from build123d import *

# Parameters (mm, degrees)
SKETCH2_R           = 50
BOSS_EXTRUDE1_DEPTH = 3
SKETCH3_R           = 6
BOSS_EXTRUDE2_DEPTH = 38.1
FILLET1_R           = 6
CUT_EXTRUDE1_DEPTH  = 38.1
SKETCH7_R           = 1.1
CUT_EXTRUDE2_DEPTH  = 2.2
SKETCH8_R           = 1.5
CUT_EXTRUDE3_DEPTH  = 3


with BuildPart() as part:
    # Sketch2 → Boss-Extrude1 (new body)
    with BuildSketch(Plane(origin=(0, 0, 0), x_dir=(1, 0, 0), z_dir=(0, 1, 0))):
        with Locations(Location((0, 0, 0), (0, 0, 270))):
            Circle(SKETCH2_R)
    extrude(amount=BOSS_EXTRUDE1_DEPTH)

    # Sketch3 → Boss-Extrude2 (add)
    with BuildSketch(Plane(origin=(0, 3, 0), x_dir=(1, 0, 0), z_dir=(0, 1, 0))):
        with Locations(Location((0, 35, 0), (0, 0, 90))):
            Circle(SKETCH3_R)
    extrude(amount=BOSS_EXTRUDE2_DEPTH)

    # Fillet1
    fillet1_edges = [part.edges().sort_by_distance(p)[0] for p in [
        (0, 41.1, -29),
    ]]
    fillet(fillet1_edges, radius=FILLET1_R)

    # Sketch6 → Cut-Extrude1 (cut)
    with BuildSketch(Plane(origin=(0, 3, 0), x_dir=(1, 0, 0), z_dir=(0, 1, 0))):
        Polygon((-43.65, 24.386010334), (-43.65, -24.386010334), (-50, -24.386010334), (-50, 0), (-50, 24.386010334), align=None)
        Polygon((43.65, 24.386010334), (43.65, -24.386010334), (50, -24.386010334), (50, 0), (50, 24.386010334), align=None)
    extrude(amount=-CUT_EXTRUDE1_DEPTH, mode=Mode.SUBTRACT)

    # Sketch7 → Cut-Extrude2 (cut)
    with BuildSketch(Plane(origin=(0, 3, 0), x_dir=(1, 0, 0), z_dir=(0, 1, 0))):
        with Locations(Location((-28.93, 11.280989666, 0), (0, 0, 270))):
            Circle(SKETCH7_R)
        with Locations(Location((-18.77, 11.280989666, 0), (0, 0, 270))):
            Circle(SKETCH7_R)
        with Locations(Location((19.07, 11.280989666, 0), (0, 0, 270))):
            Circle(SKETCH7_R)
        with Locations(Location((29.23, 11.280989666, 0), (0, 0, 270))):
            Circle(SKETCH7_R)
        with Locations(Location((29.23, -32.153010334, 0), (0, 0, 270))):
            Circle(SKETCH7_R)
        with Locations(Location((19.07, -32.153010334, 0), (0, 0, 270))):
            Circle(SKETCH7_R)
        with Locations(Location((-18.77, -32.153010334, 0), (0, 0, 270))):
            Circle(SKETCH7_R)
        with Locations(Location((-28.93, -32.153010334, 0), (0, 0, 270))):
            Circle(SKETCH7_R)
    extrude(amount=-CUT_EXTRUDE2_DEPTH, mode=Mode.SUBTRACT)

    # Sketch8 → Cut-Extrude3 (cut)
    with BuildSketch(Plane(origin=(0, 0, 0), x_dir=(-1, 0, 0), z_dir=(0, -1, 0))):
        with Locations(Location((-19.5, -26.373989666, 0), (0, 0, 90))):
            Circle(SKETCH8_R)
        with Locations(Location((8.5, -26.373989666, 0), (0, 0, 90))):
            Circle(SKETCH8_R)
        with Locations(Location((-24.5, 24.126010334, 0), (0, 0, 90))):
            Circle(SKETCH8_R)
        with Locations(Location((24.5, 24.126010334, 0), (0, 0, 90))):
            Circle(SKETCH8_R)
    extrude(amount=-CUT_EXTRUDE3_DEPTH, mode=Mode.SUBTRACT)


solid = part.part
Verification items for the finished model (mm, model axes). A direction names the side the tool comes from. Give positions to 0.01 mm unless a question says otherwise; leave off trailing zeros. Order: outer loops, then holes, each group sorted by start corner. A loop starts at its lowest first (then second) coordinate and runs counter-clockwise, first axis right, second up. Notation, with made-up numbers: M -7,-15.5 L -2,-15.5 A10 cw -2,3.5 Z; hole C -17,-29 d6. An arc over 180 degrees is marked long. Use one line per item in the form item = value. Start each with the question number.
Q1. Section check B-B (x = -24.5). Enter the section's corners in (y, z), then the cut area to 3 significant figures.
Q2. Section check D-D (y = 18). Enter the section's corners in (x, z), then the cut area to 3 significant figures.
Q3. Section check A-A (x = 0). Enter the section's corners in (y, z), then the cut area to 3 significant figures.
Q4. Scan lines: line 1 along Z through (x, y) = (19, 1); line 2 along Y through (x, z) = (-25.5, -19.5); line 3 along Z through (x, y) = (29, 1). Record each from-to range of solid material in increasing order. Write a range as [from, to].
Q5. Access from +Z, -Z, +X, -X, +Y, -Y to the whole of each face (thin tool, end or side, straight path). Record for faces 5 (the flat face through (19, 0.8, 32)), 6 (the flat face through (43.65, 2, 0)).
Q6. Mould release check, pull along X, two halves, no side actions. Record for faces 1 (the cylindrical face through (28.156, 1.915, 31.915)), 2 (the cylindrical face through (0.743, 1.479, -49.994)), 3 (the flat face through (1, 0, -1)), 4 (the flat face through (19, 0.8, -11)): +X half, -X half, draft (parallel to the pull), parting line (faces both ways), or undercut.
Q7. Go/stop test with flat-tipped pins: pin 1 Ø1.8 at (x, z) = (29.5, 32.5) entering from +Y; pin 2 Ø2.5 at (x, z) = (-24.5, -24.13) entering from -Y; pin 3 Ø1.3 at (x, z) = (19.07, 32.15) entering from +Y; pin 4 Ø5 at (y, z) = (31.5, -37.5) entering from -X. Record where each tip stops, or that it passes through.
Q8. Section check C-C (z = -14). Enter the section's corners in (x, y), then the cut area to 3 significant figures.
Evaluation:
q1.outline = M 0,-43.59 L 3,-43.59 L 3,-25.63 L 0,-25.63 Z; M 0,-22.63 L 3,-22.63 L 3,43.59 L 0,43.59 Z
q1.area = 253 mm2
q2.outline = C 0,-35 d12
q2.area = 113 mm2
q3.outline = M 0,-50 L 3,-50 L 3,-41 L 35.1,-41 A6 ccw 35.1,-29 L 3,-29 L 3,50 L 0,50 Z
q3.area = 742 mm2
q4.line_1 = [-46.25, -12.38], [-10.18, 24.96], [27.79, 31.06], [33.25, 46.25]
q4.line_2 = [0, 3]
q4.line_3 = [-40.73, -12.36], [-10.21, 31.08], [33.23, 40.73]
q5.face_5 = +Y
q5.face_6 = +Z, -Z, +X, +Y, -Y
q6.face_1 = undercut
q6.face_2 = parting line
q6.face_3 = draft
q6.face_4 = undercut
q7.pin_1 = 3
q7.pin_2 = through
q7.pin_3 = 0.8
q7.pin_4 = -6
q8.outline = M -43.65,0 L 43.65,0 L 43.65,3 L -43.65,3 Z
q8.area = 262 mm2
